```python
from build123d import *

# Parameters (mm, degrees)
CROQUIS1_R              = 4
SALIENTE_EXTRUIR1_DEPTH = 19.5
CROQUIS2_R              = 6
SALIENTE_EXTRUIR2_DEPTH = 10
CROQUIS3_R              = 4
CORTAR_EXTRUIR1_DEPTH   = 8
CORTAR_EXTRUIR2_DEPTH   = 33.407560846


with BuildPart() as part:
    # Croquis1 → Saliente-Extruir1 (new, symmetric)
    with BuildSketch(Plane.XY):
        Circle(CROQUIS1_R)
    extrude(amount=SALIENTE_EXTRUIR1_DEPTH, both=True)

    # Croquis2 → Saliente-Extruir2 (add)
    with BuildSketch(Plane.XY.offset(19.5)):
        Circle(CROQUIS2_R)
    saliente_extruir2 = extrude(amount=SALIENTE_EXTRUIR2_DEPTH)

    # Croquis3 → Cortar-Extruir1 (cut)
    with BuildSketch(Plane.XY.offset(29.5)):
        Circle(CROQUIS3_R)
    cortar_extruir1 = extrude(amount=-CORTAR_EXTRUIR1_DEPTH, mode=Mode.SUBTRACT)

    # Croquis4 → Cortar-Extruir2 (cut, through all)
    with BuildSketch(Plane(origin=(6, 0, 0), x_dir=(0, 0, -1), z_dir=(1, 0, 0))):
        with BuildLine():
            Line((-29.5, 1.25), (-23.5, 1.25))
            ThreePointArc((-23.5, 1.25), (-22.25, 0), (-23.5, -1.25))
            Line((-23.5, -1.25), (-29.5, -1.25))
            ThreePointArc((-29.5, -1.25), (-30.75, 0), (-29.5, 1.25))
        make_face()
    cortar_extruir2 = extrude(amount=-CORTAR_EXTRUIR2_DEPTH, mode=Mode.SUBTRACT)

    # Simetría2: Saliente-Extruir2, Cortar-Extruir1, Cortar-Extruir2 across plane
    add(saliente_extruir2.mirror(Plane.XY))
    add(cortar_extruir1.mirror(Plane.XY), mode=Mode.SUBTRACT)
    add(cortar_extruir2.mirror(Plane.XY), mode=Mode.SUBTRACT)


solid = part.part
```
Can you work these out from the model? Positions are in its coordinate system, mm. A direction names the side the tool comes from. Coordinates: 2 decimals unless noted, no trailing zeros. Loops run counter-clockwise (first coordinate to the right, second up) from the corner with the lowest first, then second, coordinate; pieces in that order, holes last. Notation, with made-up numbers: (-15, -33) -> (15, -33) arc R30 ccw to (15, -9) -> close; hole circle Ø4 at (-20.75, 72). An arc over 180 degrees is marked (long way). Answer as a JSON object with one key per item and string values.
1) Imagine slicing it at B-B (x = 0). Please give me the cut outline in (y, z).
Results:
{"outline": "(-6, -29.5) -> (-4, -29.5) -> (-4, -21.5) -> (4, -21.5) -> (4, -29.5) -> (6, -29.5) -> (6, -19.5) -> (4, -19.5) -> (4, 19.5) -> (6, 19.5) -> (6, 29.5) -> (4, 29.5) -> (4, 21.5) -> (-4, 21.5) -> (-4, 29.5) -> (-6, 29.5) -> (-6, 19.5) -> (-4, 19.5) -> (-4, -19.5) -> (-6, -19.5) -> close"}
2) For faces 1 (the face through (-1.42, -3.92, 19.5)), 2 (the face through (0, 0, 21.5)), 3 (the face through (-5, -1.25, 26)), 4 (the face through (-5, 1.25, -27)), which set-ups out of +Z, -Z, +X, -X, +Y, -Y let a thin tool reach every point of the face, with its end or its side?
Results:
{"face 1": "none", "face 2": "+Z", "face 3": "+Z, +X, -X", "face 4": "-Z, +X, -X"}
3) Thinking about a two-plate mould opening in Y: for faces 5 (the face through (-0.1, 4.2, -29.5)), 6 (the face through (5.54, -2.3, -24.43)), 7 (the face through (-5, -1.25, -26)), which applies, pulls with the +Y half, pulls with the -Y half, needs draft (parallel to the pull), parting line crosses it, or undercut?
Results:
{"face 5": "needs draft", "face 6": "parting line crosses it", "face 7": "undercut"}
4) If I drill on line 1 (Z direction, x = 0.5, y = 5.25); line 2 (Y direction, x = 0, z = -25.75); line 3 (X direction, y = 2.5, z = -23), over which ranges is the centre line in solid material (lowest first)?
Results:
{"line 1": "z = -29.5 to -19.5, 19.5 to 29.5", "line 2": "y = -6 to -4, 4 to 6", "line 3": "x = -5.45 to -3.12, 3.12 to 5.45"}
5) Imagine slicing it at D-D (y = -4.75). Please give me the cut outline in (x, z), then the cut area to 3 significant figures.
Results:
{"outline": "(-3.67, -29.5) -> (3.67, -29.5) -> (3.67, -19.5) -> (-3.67, -19.5) -> close; (-3.67, 19.5) -> (3.67, 19.5) -> (3.67, 29.5) -> (-3.67, 29.5) -> close", "area": "147 mm^2"}
6) Imagine slicing it at A-A (z = -25.5). Please give me the cut outline in (x, y).
Results:
{"outline": "(-5.87, -1.25) arc R6 ccw to (5.87, -1.25) -> (3.8, -1.25) arc R4 cw to (-3.8, -1.25) -> close; (-5.87, 1.25) -> (-3.8, 1.25) arc R4 cw to (3.8, 1.25) -> (5.87, 1.25) arc R6 ccw to start"}
7) For P1, Ø3, axis at x = -0.5, z = -4, coming from the -Y side; P2, Ø1, axis at x = 1.5, z = 13.5, coming from the +Y side; P3, Ø6.5, axis at x = 0, y = 0, coming from the +Z side, each with a flat end and sliding along its axis, tell me the tip position at first contact or that it passes through.
Results:
{"P1": "stops at y = -4", "P2": "stops at y = 3.87", "P3": "stops at z = 21.5"}
8) Imagine slicing it at C-C (y = 0). Please give me the cut outline in (x, z).
Results:
{"outline": "(-6, -22.25) -> (-4, -22.25) -> (-4, -21.5) -> (4, -21.5) -> (4, -22.25) -> (6, -22.25) -> (6, -19.5) -> (4, -19.5) -> (4, 19.5) -> (6, 19.5) -> (6, 22.25) -> (4, 22.25) -> (4, 21.5) -> (-4, 21.5) -> (-4, 22.25) -> (-6, 22.25) -> (-6, 19.5) -> (-4, 19.5) -> (-4, -19.5) -> (-6, -19.5) -> close"}
